Here's the drawing with two shaded views (mm, measured from the low corner). I have some questions. A direction names the side the tool comes from. Give positions to 0.01 mm unless a question says otherwise; leave off trailing zeros. Write each loop counter-clockwise with the first axis right and the second up, starting at its lowest first coordinate (ties: lowest second). Pieces come first, ordered by that corner, then holes.
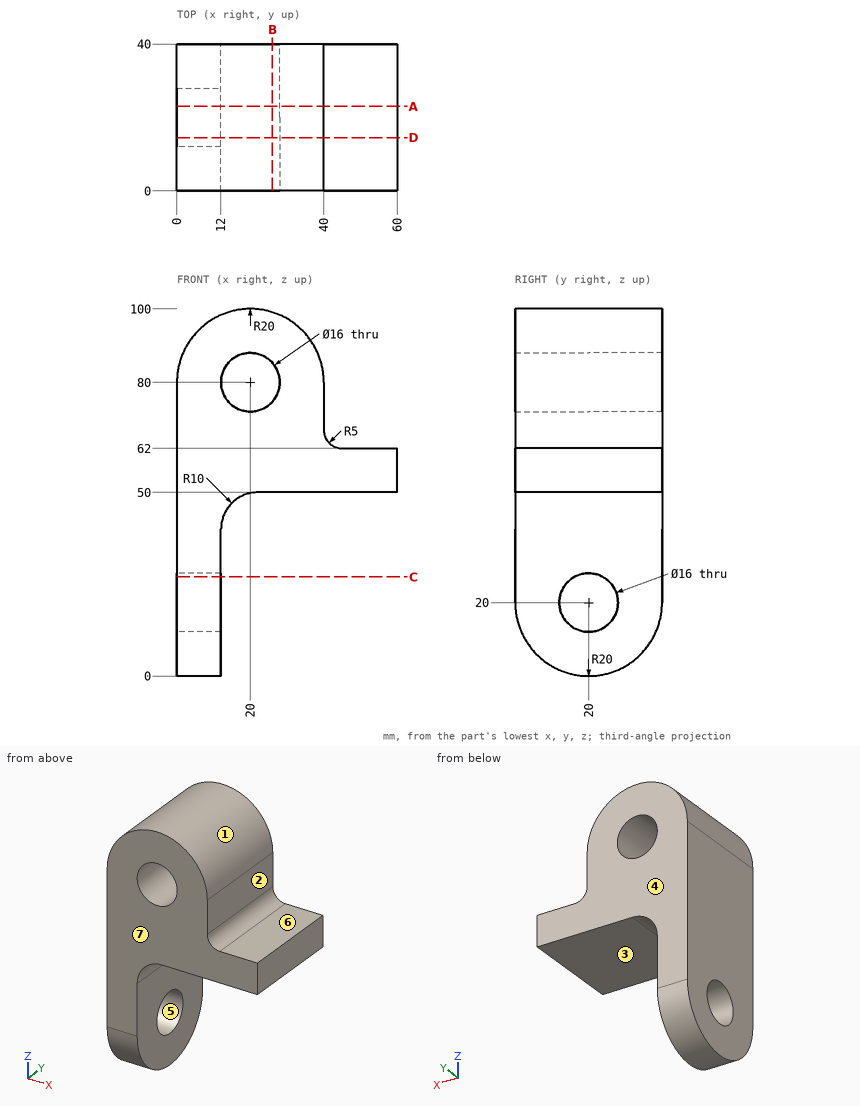
(1) If we mould it in two halves opening along Y, with no side actions, what happens to the marked faces 4, 5, 6 and 7? For each: +Y half, -Y half, draft (parallel to the pull), parting line (faces both ways), or undercut.
Returned:
face 4: +Y half
face 5: undercut
face 6: draft
face 7: -Y half
(2) For the marked faces 1, 2 and 3, which set-ups out of +Z, -Z, +X, -X, +Y, -Y let a thin tool reach every point of the face, with its end or its side?
Returned:
face 1: +Z, +Y, -Y
face 2: +Z, +X, +Y, -Y
face 3: -Z, +X, +Y, -Y
(3) Imagine slicing it at A-A, the plane y = 23. Write out the boundary of the cut face in (x, z), plus the area to 3 significant figures.
Returned:
outline: (0, 0.23) - (12, 0.23) - (12, 12.58) - (0, 12.58) - close; (0, 27.42) - (12, 27.42) - (12, 40) arc R10 cw to (22, 50) - (60, 50) - (60, 62) - (45, 62) arc R5 cw to (40, 67) - (40, 80) arc R20 ccw to (0, 80) - close; hole circle Ø16 at (20, 80)
area: 2,310 mm2
(4) Imagine slicing it at D-D, the plane y = 14.5. Write out the boundary of the cut face in (x, z).
Returned:
outline: (0, 0.77) - (12, 0.77) - (12, 14.19) - (0, 14.19) - close; (0, 25.81) - (12, 25.81) - (12, 40) arc R10 cw to (22, 50) - (60, 50) - (60, 62) - (45, 62) arc R5 cw to (40, 67) - (40, 80) arc R20 ccw to (0, 80) - close; hole circle Ø16 at (20, 80)
(5) If I drill on L1, parallel to X at y = 11, z = 80; L2, parallel to Z at x = 24.5, y = 30.5, over which ranges is the centre line in solid material (lowest first)?
Returned:
L1: x = 0 to 12, 28 to 40
L2: z = 50 to 73.39, 86.61 to 99.49
(6) Imagine slicing it at B-B, the plane x = 26. Write out the boundary of the cut face in (y, z).
Returned:
outline: (0, 50) - (40, 50) - (40, 74.71) - (0, 74.71) - close; (0, 85.29) - (40, 85.29) - (40, 99.08) - (0, 99.08) - close
(7) Will these pins go through, and if not, where does the flat tip stop? P1, Ø7.5, axis at x = 50, y = 26.5, coming from the +Z side; P2, Ø3, axis at y = 34.5, z = 18, coming from the -X side; P3, Ø8, axis at y = 7, z = 75.5, coming from the +X side; P4, Ø6, axis at y = 22, z = 15, coming from the +X side.
Returned:
P1: stops at z = 62
P2: stops at x = 0
P3: stops at x = 40
P4: stops at x = 12
(8) Imagine slicing it at C-C, the plane z = 27. Write out the boundary of the cut face in (x, y).
Returned:
outline: (0, 0) - (12, 0) - (12, 16.13) - (0, 16.13) - close; (0, 23.87) - (12, 23.87) - (12, 40) - (0, 40) - close
